The model under review builds one solid part; all positions refer to its coordinate system, in mm. Coordinates: 2 decimals unless noted, no trailing zeros. Order: outer loops, then holes, each group sorted by start corner. A loop starts at its lowest first (then second) coordinate and runs counter-clockwise, first axis right, second up. Notation, with made-up numbers: M 48.5,-35.5 L 106.5,-35.5 A11 ccw 106.5,-15.5 Z; hole C 3,57.25 d4. An arc over 180 degrees is marked long. One line per item, written item: value.
```python
from build123d import *

# Parameters (mm, degrees)
SKETCH_1_W      = 100
SKETCH_1_H      = 15
SKETCH_1_R      = 3
EXTRUDE_1_DEPTH = 3


with BuildPart() as part:
    # Эскиз1 → Бобышка-Вытянуть1 (new body)
    with BuildSketch(Plane(origin=(0, 0, 0), x_dir=(0, 0, -1), z_dir=(1, 0, 0))):
        Rectangle(SKETCH_1_W, SKETCH_1_H)
        with Locations((-40, 0)):
            Circle(SKETCH_1_R, mode=Mode.SUBTRACT)
        with Locations((-20, 0)):
            Circle(SKETCH_1_R, mode=Mode.SUBTRACT)
        with Locations(Location((20, 0, 0), (0, 0, 180))):
            Circle(SKETCH_1_R, mode=Mode.SUBTRACT)
        with Locations(Location((40, 0, 0), (0, 0, 180))):
            Circle(SKETCH_1_R, mode=Mode.SUBTRACT)
    extrude(amount=EXTRUDE_1_DEPTH)


solid = part.part
```
(1) We need section D-D, the plane z = 21.5. State the section outline as (x, y) points.
Geometry results:
outline: M 0,-7.5 L 3,-7.5 L 3,-2.6 L 0,-2.6 Z; M 0,2.6 L 3,2.6 L 3,7.5 L 0,7.5 Z
(2) We need section A-A, the plane y = 0. State the section outline as (x, z) points.
Geometry results:
outline: M 0,-50 L 3,-50 L 3,-43 L 0,-43 Z; M 0,-37 L 3,-37 L 3,-23 L 0,-23 Z; M 0,-17 L 3,-17 L 3,17 L 0,17 Z; M 0,23 L 3,23 L 3,37 L 0,37 Z; M 0,43 L 3,43 L 3,50 L 0,50 Z
(3) Mouldability with a two-part tool opening along Z and no side actions: class faces 1 (the flat face through (1, 0, 50)), 2 (the cylindrical face through (1, 0, -23)), 3 (the flat face through (1, -7.5, 1)) as +Z half, -Z half, draft (parallel to the pull), parting line (faces both ways), or undercut.
Geometry results:
face 1: +Z half
face 2: undercut
face 3: draft
(4) We need section C-C, the plane x = 1.7. State the section outline as (y, z) points, plus the area to 3 significant figures.
Geometry results:
outline: M -7.5,-50 L 7.5,-50 L 7.5,50 L -7.5,50 Z; hole C 0,-40 d6; hole C 0,-20 d6; hole C 0,20 d6; hole C 0,40 d6
area: 1,390 mm2
(5) We need section B-B, the plane z = -40. State the section outline as (x, y) points, plus the area to 3 significant figures.
Geometry results:
outline: M 0,-7.5 L 3,-7.5 L 3,-3 L 0,-3 Z; M 0,3 L 3,3 L 3,7.5 L 0,7.5 Z
area: 27.0 mm2
(6) For L1, parallel to Y at x = 0.8, z = -20; L2, parallel to Y at x = 1.9, z = 17.5; L3, parallel to Z at x = 0.5, y = 1.75, list the stretches that pass through material, from the lowest coordinate up.
Geometry results:
L1: y = -7.5 to -3, 3 to 7.5
L2: y = -7.5 to -1.66, 1.66 to 7.5
L3: z = -50 to -42.44, -37.56 to -22.44, -17.56 to 17.56, 22.44 to 37.56, 42.44 to 50
